Design review of the part built by this model. Coordinates are the model's own, in mm. A direction names the side the tool comes from. Coordinates: 2 decimals unless noted, no trailing zeros. Loops run counter-clockwise (first coordinate to the right, second up) from the corner with the lowest first, then second, coordinate; pieces in that order, holes last. Notation, with made-up numbers: (-32.75, -5.75) -> (-15.75, -5.75) arc R11 cw to (-15.75, 10.25) -> close; hole circle Ø10 at (-17, 75.25). An arc over 180 degrees is marked (long way). Answer as a JSON object with one key per item and string values.
Autodesk Inventor part; units mm, degrees
ref_plane "YZ Plane" through (0, 0, 0) normal (1, 0, 0) x (0, 1, 0)
ref_plane "XZ Plane" through (0, 0, 0) normal (0, 1, 0) x (-1, 0, 0)
ref_plane "XY Plane" through (0, 0, 0) normal (0, 0, 1) x (1, 0, 0)
sketch "スケッチ1" plane through (0, 0, 0) normal (0, 0, 1) x (1, 0, 0)
  line L0 (-16.5, 13) -> (16.5, 13)
  line L1 (16.5, 13) -> (16.5, -13)
  line L2 (16.5, -13) -> (-16.5, -13)
  line L3 (-16.5, -13) -> (-16.5, 13)
  line L4 (-16.5, 13) -> (16.5, -13) construction
  line L5 (16.5, 13) -> (-16.5, -13) construction
  circle A0 centre (0, 0) radius 10
  dimension "d0" = 33
  dimension "d1" = 26
  dimension "d2" = 20
extrude "押し出し1" add sketch "スケッチ1" along normal blind 70
sketch "スケッチ2" plane through (-16.5, -13, 0) normal (0, -1, 0) x (1, 0, 0)
  line L0 (18.5, 60) -> (18.5, 0)
  line L1 (18.5, 0) -> (14.5, 0)
  line L2 (14.5, 0) -> (14.5, 60)
  line L3 (18.5, 70) -> (14.5, 0) construction
  line L4 (18.5, 0) -> (14.5, 70) construction
  line L5 (0, 0) -> (33, 0)
  line L6 (18.5, 60) -> (14.5, 60)
  point P0 (16.5, 0)
  point P1 (16.5, 35)
  dimension "d5" = 4
extrude "押し出し2" cut sketch "スケッチ2" against normal blind 50
sketch "スケッチ3" plane through (0, 0, 70) normal (0, 0, 1) x (1, 0, 0)
  line L0 (-16.5, -13) -> (16.5, -13)
  line L1 (16.5, -13) -> (16.5, 13)
  line L2 (16.5, 13) -> (-16.5, 13)
  circle A0 centre (0, 0) radius 10
  circle A1 centre (0, 0) radius 10
  line L3 (16.5, 13) -> (-16.5, 13)
  line L4 (-16.5, 13) -> (-16.5, -13)
  line L5 (-16.5, -13) -> (16.5, -13)
  line L6 (16.5, -13) -> (-16.5, -13)
  line L7 (-16.5, -13) -> (-16.5, 13)
  line L8 (-16.5, 13) -> (16.5, 13)
  line L9 (16.5, 13) -> (16.5, -13)
  circle A2 centre (0, 0) radius 10
  line L10 (16.5, -13) -> (16.5, 13)
  line L11 (-16.5, 13) -> (-16.5, -13)
  dimension "d8" = 20
extrude "押し出し3" add sketch "スケッチ3" along normal blind 5
sketch "スケッチ4" plane through (0, 0, 0) normal (0, 0, -1) x (-1, 0, 0)
  line L0 (30, -4) -> (30, 4)
  line L1 (-30, 4) -> (-30, -4)
  line L2 (-30, -4) -> (30, 4) construction
  line L3 (30, -4) -> (-30, 4) construction
  line L4 (-2, 13) -> (-16.5, 13)
  line L5 (-16.5, 13) -> (-30, 4)
  line L6 (-16.5, 13) -> (-16.5, -13)
  line L7 (-30, -4) -> (-16.5, -13)
  line L8 (2, -9.798) -> (2, -13)
  line L9 (2, -13) -> (16.5, -13)
  line L10 (16.5, -13) -> (16.5, 13)
  line L11 (16.5, 13) -> (2, 13)
  line L12 (2, 13) -> (2, 9.798)
  arc A0 (2, -9.798) -> (2, 9.798) centre (0, 0) ccw
  line L13 (-2, -13) -> (-2, -9.798)
  arc A1 (-2, 9.798) -> (-2, -9.798) centre (0, 0) ccw
  line L14 (-2, 9.798) -> (-2, 13)
  line L15 (-2, 13) -> (-16.5, 13)
  line L16 (-16.5, 13) -> (-16.5, -13)
  line L17 (-16.5, -13) -> (-2, -13)
  line L18 (16.5, -13) -> (30, -4)
  line L19 (30, 4) -> (16.5, 13)
  circle A2 centre (-23.25, 0) radius 1.75
  circle A3 centre (23.25, 0) radius 1.75
  dimension "d15" = 3.5
  dimension "d16" = 3.5
extrude "押し出し4" add sketch "スケッチ4" against normal blind 8 contours L18 L10 L19 L0 | L5 L6 L7 L1
chamfer "面取り1" distance 2 angle 45 10 edges at (16.5, 0, 8) (-16.5, 0, 8) (16.5, -13, 41.5) (16.5, 13, 41.5) (-16.5, -13, 41.5) (-16.5, -13, 4) (16.5, -13, 4) (-16.5, 13, 41.5) (-16.5, 13, 4) (16.5, 13, 4)
properties part number "RescueKit-Pipev2"
1) Add section A-A, the plane z = 32. Give the boundary of the cut face in (x, y), and give its area (3 significant figures).
Completed:
{"outline": "(-16.5, -11) -> (-14.5, -13) -> (-2, -13) -> (-2, -9.8) arc R10 cw to (-2, 9.8) -> (-2, 13) -> (-14.5, 13) -> (-16.5, 11) -> close; (2, -13) -> (14.5, -13) -> (16.5, -11) -> (16.5, 11) -> (14.5, 13) -> (2, 13) -> (2, 9.8) arc R10 cw to (2, -9.8) -> close", "area": "511 mm²"}
2) Add section D-D, the plane y = 6. Give the boundary of the cut face in (x, z), and give its area (3 significant figures).
Completed:
{"outline": "(-27, 0) -> (-8, 0) -> (-8, 75) -> (-16.5, 75) -> (-16.5, 10) -> (-18.5, 8) -> (-27, 8) -> close; (8, 0) -> (27, 0) -> (27, 8) -> (18.5, 8) -> (16.5, 10) -> (16.5, 75) -> (8, 75) -> close", "area": "1,450 mm²"}
3) For faces 1 (the flat face through (-16.5, 0, 42)), 2 (the flat face through (17.5, 0.2, 9)), 3 (the flat face through (2, 11, 30)), list the 3-axis set-ups (+Z, -Z, +X, -X, +Y, -Y) from which the entire face can be reached by the end or side of a thin tool; tool diameter is ignored.
Completed:
{"face 1": "+Z, -X, +Y, -Y", "face 2": "+Z, +X, +Y, -Y", "face 3": "-Z, +Y, -Y"}
4) Clearance check with flat-ended pins moving along their axes: pin 1 Ø2 at (y, z) = (1.5, 47) entering from +X; pin 2 Ø1.6 at (y, z) = (-10.5, 23.5) entering from -X; pin 3 Ø1 at (y, z) = (12, 29.5) entering from +X; pin 4 Ø4 at (x, z) = (16, 64.5) entering from -Y. State where each tip first meets the part, or that it passes through.
Completed:
{"pin 1": "x = 16.5", "pin 2": "x = -16.5", "pin 3": "x = 16", "pin 4": "y = -13"}
5) Wall thickness on probe 1 along X at (y, z) = (10, 56.5); probe 2 along Y at (x, z) = (-8.5, 24.5); probe 3 along X at (y, z) = (-8.25, 27): over which ranges is each line inside the solid? List them lowest first.
Completed:
{"probe 1": "-16.5 to -2, 2 to 16.5", "probe 2": "-13 to -5.27, 5.27 to 13", "probe 3": "-16.5 to -5.65, 5.65 to 16.5"}
6) Add section C-C, the plane y = 0. Give the boundary of the cut face in (x, z).
Completed:
{"outline": "(-30, 0) -> (-25, 0) -> (-25, 8) -> (-30, 8) -> close; (-21.5, 0) -> (-10, 0) -> (-10, 75) -> (-16.5, 75) -> (-16.5, 10) -> (-18.5, 8) -> (-21.5, 8) -> close; (10, 0) -> (21.5, 0) -> (21.5, 8) -> (18.5, 8) -> (16.5, 10) -> (16.5, 75) -> (10, 75) -> close; (25, 0) -> (30, 0) -> (30, 8) -> (25, 8) -> close"}
7) The part is to be moulded in two halves that separate along X. For faces 4 (the flat face through (0, -11, 60)), 5 (the flat face through (-15.6, -11.9, 41)), 6 (the flat face through (15.6, -11.9, 41)), say which applies: pulls with the +X half, pulls with the -X half, needs draft (parallel to the pull), parting line crosses it, or undercut.
Completed:
{"face 4": "undercut", "face 5": "pulls with the -X half", "face 6": "pulls with the +X half"}
8) Add section B-B, the plane x = -23.25. Give the boundary of the cut face in (y, z), and give its area (3 significant figures).
Completed:
{"outline": "(-8.5, 0) -> (-1.75, 0) -> (-1.75, 8) -> (-8.5, 8) -> close; (1.75, 0) -> (8.5, 0) -> (8.5, 8) -> (1.75, 8) -> close", "area": "108 mm²"}
